Autodesk Inventor part; units mm, degrees
ref_plane "YZ Plane" through (0, 0, 0) normal (1, 0, 0) x (0, 1, 0)
ref_plane "XZ Plane" through (0, 0, 0) normal (0, 1, 0) x (-1, 0, 0)
ref_plane "XY Plane" through (0, 0, 0) normal (0, 0, 1) x (1, 0, 0)
sketch "Sketch1" plane through (0, 0, 0) normal (0, 0, 1) x (1, 0, 0)
  circle A0 centre (0, 0) radius 6.75
  dimension "d0" = 13.5
extrude "Extrusion1" add sketch "Sketch1" along normal blind 11.315
sketch "Sketch2" plane through (0, 0, 11.315) normal (0, 0, 1) x (1, 0, 0)
  arc A0 (0, -6.75) -> (0, 6.75) centre (0, 0) ccw
  line L0 (0, 6.75) -> (0, -6.75)
revolve "Revolution1" add sketch "Sketch2" angle 360 about axis through (0, 6.75, 11.315) along (0, -1, 0)
sketch "Sketch3" plane through (0, 0, 0) normal (1, 0, 0) x (0, 1, 0)
  line L0 (6.9939, 18.3652) -> (6.9939, -0.2867) construction
  line L1 (6.9939, -0.2867) -> (-6.6981, -0.2867) construction
  line L2 (-6.6981, -0.2867) -> (-6.6981, 18.3652) construction
  line L3 (-6.6981, 18.3652) -> (6.9939, 18.3652) construction
  line L4 (7.5187, 2.3916) -> (5.1843, 6.3459)
  spline S0 degree 3 poles (2.2232, 17.6743) (3.9137, 15.2739) (5.2905, 10.1216) (5.1843, 6.3459) knots 0 0 0 0 1 1 1 1
  spline S1 degree 4 poles (-2.7095, 17.5553) (-3.4345, 16.3323) (-3.9815, 15.3648) (-4.6404, 13.6169) (-5.2893, 11.6954) (-5.7416, 9.7633) (-6.0904, 7.9156) (-6.2555, 6.3812) (-6.4601, 3.9007) (-6.437, 2.3154) (-6.3311, 0.3242) (-6.2339, -0.1725) knots 0 0 0 0 0 0.226948 0.315631 0.407822 0.501079 0.595945 0.688744 0.781622 1 1 1 1 1
  arc A0 (2.2232, 17.6743) -> (-2.7095, 17.5553) centre (-0.2549, 18.1011) ccw
  line L5 (7.5187, 2.3916) -> (7.6074, -3.0566)
  line L6 (7.6074, -3.0566) -> (-6.5982, -2.034)
  line L7 (-6.5982, -2.034) -> (-6.1989, -0.3494)
  line L8 (-6.1989, -0.3494) -> (-6.2339, -0.1725)
  line L9 (-10.6943, 22.9274) -> (9.6594, 22.9274)
  line L10 (9.6594, 22.9274) -> (9.6594, -5.6031)
  line L11 (9.6594, -5.6031) -> (-10.6943, -5.6031)
  line L12 (-10.6943, -5.6031) -> (-10.6943, 22.9274)
  line L13 (-10.6943, 22.9274) -> (9.6594, -5.6031) construction
  line L14 (9.6594, 22.9274) -> (-10.6943, -5.6031) construction
  point P0 (0, 0)
  point P1 (3.606, 14.941)
  point P2 (4.8031, 10.6278)
  point P3 (-3.6969, 15.797)
  point P4 (-4.2759, 14.5167)
  point P5 (-4.7839, 13.1635)
  point P6 (-5.2449, 11.7299)
  point P7 (-5.7181, 9.7886)
  point P8 (-6.0639, 7.9039)
  point P9 (-6.252, 6.3205)
  point P10 (-6.3835, 4.5875)
  point P11 (-6.4199, 2.9071)
  point P12 (-6.3492, 0.98)
  point P13 (-0.5174, 8.6621)
extrude "Extrusion2" cut sketch "Sketch3" against normal mid plane 15.315
sketch "Sketch4" plane through (0, 0, 0) normal (1, 0, 0) x (0, 1, 0)
  line L0 (0, 0) -> (4.875, 0)
  line L1 (6.75, 0) -> (-6.2616, 0)
  line L2 (4.875, 0) -> (4.875, 1.45)
  line L3 (4.875, 1.45) -> (5.56, 1.45)
  line L4 (5.56, 1.45) -> (5.56, 2.95)
  line L5 (5.56, 2.95) -> (5.56, 4.2347)
  line L6 (3.91, 4.3347) -> (5.56, 2.95)
  line L7 (0, 0) -> (0, 14.3)
  line L8 (0, 14.3) -> (3.1075, 14.3)
  line L9 (3.1075, 14.3) -> (3.91, 4.3347)
  dimension "d57" = 4.875
  dimension "d58" = 1.45
  dimension "d59" = 0.685
  dimension "d60" = 1.5
  dimension "d61" = 1.2847
  dimension "d63" = 14.3
  dimension "d64" = 3.1075
revolve "Revolution2" cut sketch "Sketch4" angle 360 about axis through (0, 0, 0) along (0, 0, 1)
properties part number "TipTip"
Geometry: final body of the model. Coordinates: model frame, mm. A direction names the side the tool comes from. Round coordinates to 2 decimals unless told otherwise and drop trailing zeros. Write each loop counter-clockwise with the first axis right and the second up, starting at its lowest first coordinate (ties: lowest second). Pieces come first, ordered by that corner, then holes.
Item 1: Section query B-B (y = 6.25). Return loops of the section in (x, z).
Item 2: Set-up query: faces 1 (the face through (0.1, 5.8, 5.3)), 2 (the face through (5, 2, 1.45)), 3 (the face through (0, 0, 14.3)). Return all of +Z, -Z, +X, -X, +Y, -Y with unobstructed straight access to the full face (end or side cutting, diameter ignored); none if empty.
Item 3: Mould query, pull axis X, two halves, no side actions, for faces 4 (the face through (4.18, -5.3, 4.32)), 5 (the face through (-2.138, -2.789, 9.248)), 6 (the face through (1, 5, 0)). Classes: +X half, -X half, draft (parallel to the pull), parting line (faces both ways), or undercut.
Item 4: Material intervals for L1, parallel to X at y = 0, z = 2.15; L2, parallel to X at y = 0, z = 0.65 (3 decimals); L3, parallel to Y at x = 2.5, z = 12, sorted ascending.
Item 5: Pin query (flat end, axial travel): P1, Ø3, axis at x = 2.5, z = 9.5, coming from the +Y side (3 decimals); P2, Ø3, axis at x = -3.5, y = 4, coming from the +Z side; P3, Ø1.5, axis at x = 0.5, z = 9.5, coming from the -Y side. Return the tip coordinate at first contact, or that it passes through.
Completed:
1. outline: (-2.55, 0) - (2.55, 0) - (2.55, 4.54) - (-2.55, 4.54) - close
2. face 1: +Z, +X, -X, +Y
2. face 2: none
2. face 3: -Z
3. face 4: parting line
3. face 5: undercut
3. face 6: draft
4. L1: x = -6.75 to -5.56, 5.56 to 6.75
4. L2: x = -6.75 to -4.875, 4.875 to 6.75
4. L3: y = -5.17 to -2.14, 2.14 to 4.51
5. P1: stops at y = 5.145
5. P2: stops at z = 16.86
5. P3: stops at y = -5.92
